Part model, mm, in its own coordinate system. Round coordinates to 2 decimals unless told otherwise and drop trailing zeros. Loops run counter-clockwise (first coordinate to the right, second up) from the corner with the lowest first, then second, coordinate; pieces in that order, holes last. Notation, with made-up numbers: M -21,85.5 L 15,85.5 A15 ccw 15,101.5 Z; hole C 15.5,15.5 d5. An arc over 180 degrees is marked long. Put each result on its own line as item: value. Start each with the question number.
1) Probe line 1 along X through (y, z) = (21.5, 0.05); line 2 along Y through (x, z) = (12.75, 0.05); line 3 along X through (y, z) = (14, 0.05). List the from-to ranges inside material, lowest first.
2) Slice it at A-A on z = 0.05. Give the cut face in (x, y), then the cut area to 3 significant figures.
3) Slice it at B-B on x = 20.5. Give the cut face in (y, z).
4) Slice it at C-C on y = 26. Give the cut face in (x, z), then the cut area to 3 significant figures.
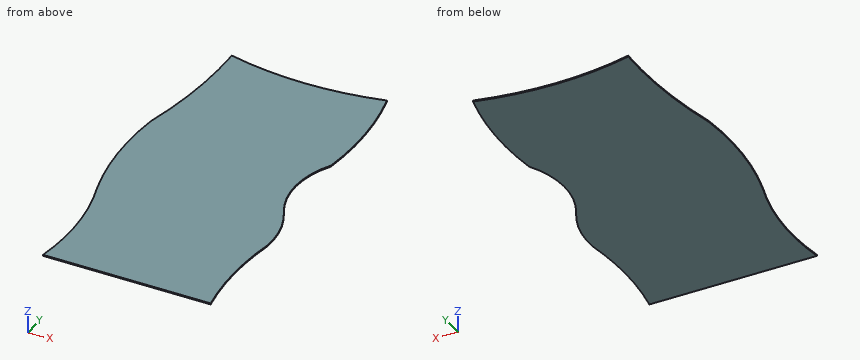
```python
from build123d import *

# Parameters (mm, degrees)
SALIENTE_EXTRUIR1_DEPTH = 0.1


with BuildPart() as part:
    # Model → Saliente-Extruir1 (new body)
    with BuildSketch(Plane.XY):
        with BuildLine():
            Line((11.080118073, 12.100032616), (26.494172291, 12.100013434))
            ThreePointArc((26.494172291, 12.100013434), (25.962033929, 17.071786447), (26.334882576, 22.058035741))
            ThreePointArc((26.334882576, 22.058035741), (26.077271745, 24.671051179), (25.080126231, 27.100025003))
            ThreePointArc((25.080126231, 27.100025003), (24.017870658, 31.10002558), (25.080130581, 35.100025003))
            ThreePointArc((25.080130581, 35.100025003), (25.229028906, 40.534712367), (24.350613381, 45.900006732))
            ThreePointArc((24.350613381, 45.900006732), (17.215374003, 45.022517475), (10.080135103, 45.900010617))
            ThreePointArc((10.080135103, 45.900010617), (9.999432675, 39.964488004), (9.080130038, 34.100033704))
            ThreePointArc((9.080130038, 34.100033704), (9.035519695, 28.550523972), (10.080124055, 23.10003316))
            ThreePointArc((10.080124055, 23.10003316), (11.257202038, 17.661585333), (11.080118073, 12.100032616))
        make_face()
    extrude(amount=SALIENTE_EXTRUIR1_DEPTH)


solid = part.part
```
Recorded:
1. line 1: x = 10.57 to 26.25
1. line 2: y = 12.1 to 45.36
1. line 3: x = 11.29 to 26.18
2. outline: M 9.08,34.1 A28.16 ccw 10.08,23.1 A22.77 cw 11.08,12.1 L 26.49,12.1 A27.62 cw 26.33,22.06 A9.05 ccw 25.08,27.1 A8.06 cw 25.08,35.1 A28.71 ccw 24.35,45.9 A29.45 cw 10.08,45.9 A41.87 cw Z
2. area: 509 mm2
3. outline: M 12.1,0 L 45.21,0 L 45.21,0.1 L 12.1,0.1 Z
4. outline: M 9.39,0 L 25.63,0 L 25.63,0.1 L 9.39,0.1 Z
4. area: 1.62 mm2
